from build123d import *

# Parameters (mm, degrees)
KOPF_DEPTH = 2.8
SKIZZE3_W  = 1.091451884
SKIZZE3_H  = 0.4
SKIZZE2_W  = 1.55
SKIZZE2_H  = 12
SKIZZE4_W  = 2.35
SKIZZE4_H  = 0.8


with BuildPart() as part:
    # Skizze1 → Kopf (new body)
    with BuildSketch(Plane(origin=(0, 0.8, 0), x_dir=(1, 0, 0), z_dir=(0, 1, 0))):
        Polygon((3.5, 2.020725942), (0, 4.041451884), (-3.5, 2.020725942), (-3.5, -2.020725942), (0, -4.041451884), (3.5, -2.020725942), align=None)
    extrude(amount=KOPF_DEPTH)

    # Skizze3 → Schnitt Kopf (revolve, cut)
    with BuildSketch(Plane(origin=(0, 0, 0), x_dir=(0, 0, -1), z_dir=(1, 0, 0))):
        Polygon((4.041451884, 3.6), (3.5, 3.6), (4.041451884, 3.381239239), align=None)
        with Locations((3.495725942, 1)):
            Rectangle(SKIZZE3_W, SKIZZE3_H)
    revolve(axis=Axis((0, 0, 0), (0, 1, 0)), mode=Mode.SUBTRACT)

    # Skizze2 → Gewinde (revolve)
    with BuildSketch(Plane.XY, mode=Mode.PRIVATE) as gewinde_sk:
        with Locations((0.775, -5.2)):
            Rectangle(SKIZZE2_W, SKIZZE2_H)
    revolve(gewinde_sk.sketch.rotate(Axis((0, 5.086887038, 0), (0, -1, 0)), 270), axis=Axis((0, 5.086887038, 0), (0, -1, 0)))  # turned: the seam where the file's is

    # Skizze4 → Rotation1 (revolve)
    with BuildSketch(Plane(origin=(0, 0, 0), x_dir=(0, 0, -1), z_dir=(1, 0, 0))):
        with Locations((3.325, 0.4)):
            Rectangle(SKIZZE4_W, SKIZZE4_H)
    revolve(axis=Axis((0, 0, 0), (0, 1, 0)))


solid = part.part
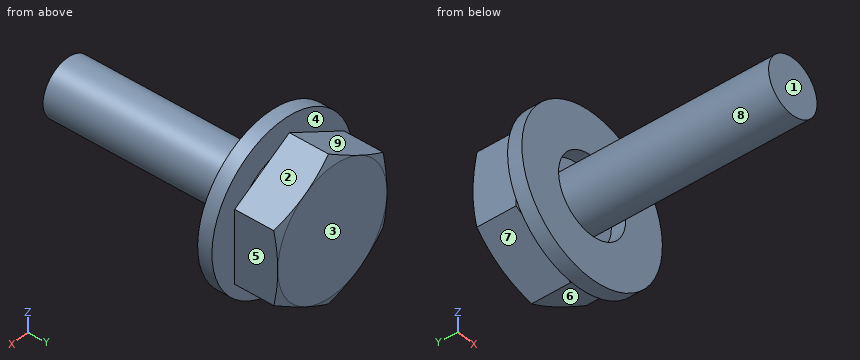
Geometry: final body of the model. Coordinates: model frame, mm. Face numbers are marked on the shaded views. A direction names the side the tool comes from. Give positions to 0.01 mm unless a question says otherwise; leave off trailing zeros. Loops run counter-clockwise (first coordinate to the right, second up) from the corner with the lowest first, then second, coordinate; pieces in that order, holes last. Notation, with made-up numbers: (11, 31.5) -> (69, 31.5) arc R17 ccw to (69, 43.5) -> close; hole circle Ø5 at (75.25, 56.5). An arc over 180 degrees is marked (long way). Put each result on its own line as item: value.
1. Pull-direction query (Y, two-part tool) for the marked faces 1, 2, 3 and 4; classes: released by +Y, released by -Y, zero draft, split by the parting line, or undercut.
Taken from the geometry:
face 1: released by -Y
face 2: zero draft
face 3: released by +Y
face 4: undercut
2. Ray query, line 1 along X through (y, z) = (0.55, 0); line 2 along Y through (x, z) = (3, -1); line 3 along Y through (x, z) = (-2.25, 3). Return the intervals inside material, ascending. Write a range as [from, to].
Taken from the geometry:
line 1: x = [-4.5, -2.15], [-1.55, 1.55], [2.15, 4.5]
line 2: y = [0, 0.8], [1.2, 3.6]
line 3: y = [0, 0.8]
3. Pin query (flat end, axial travel): P1, Ø5, axis at y = -4.5, z = 2.5, coming from the -X side; P2, Ø1.9, axis at y = 3, z = 0, coming from the -X side; P3, Ø3, axis at x = 2, y = -6.5, coming from the +Z side. Return the tip coordinate at first contact, or that it passes through.
Taken from the geometry:
P1: stops at x = -1.55
P2: stops at x = -3.5
P3: stops at z = 1.47
4. Cut plane B-B (y = -5.75). Return the cut outline in (x, z), plus the area to 3 significant figures.
Taken from the geometry:
outline: circle Ø3.1 at (0, 0)
area: 7.55 mm2
5. Set-up query: the marked faces 5, 6, 7, 8 and 9. Return all of +Z, -Z, +X, -X, +Y, -Y with unobstructed straight access to the full face (end or side cutting, diameter ignored); none if empty.
Taken from the geometry:
face 5: +Z, -Z, +X, +Y
face 6: -Z, +X, +Y
face 7: -Z, -X, +Y
face 8: -Y
face 9: +Z, -X, +Y
6. Cut plane A-A (y = 0.5). Return the cut outline in (x, z), plus the area to 3 significant figures.
Taken from the geometry:
outline: circle Ø9 at (0, 0); circle Ø3.1 at (0, 0); hole circle Ø4.3 at (0, 0)
area: 56.6 mm2
